```python
from build123d import *

# Parameters (mm, degrees)
F1_W            = 1250
F1_H            = 1250
F2_DEPTH        = 10
F0_W            = 125
F0_H            = 125
F3_DEPTH        = 0.1
F4_W            = 1270
F4_H            = 1270
F4_W_2          = 1250
F4_H_2          = 1250
F5_DEPTH        = 260
F6_W            = 125
F6_H            = 125
F7_DEPTH        = 0.1
F7_COPIES_COUNT = 3
F7_COPIES_ANGLE = 180
F9_W            = 1250
F9_H            = 10
F10_DEPTH       = 250


# Not quite as in the source:
# - a pattern or mirror of a feature is missing from the dataset's text; its kind, count and spacing are read off the source's solid


with BuildPart() as f2:
    # F1 (on Top) → F2 (new body)
    with BuildSketch(Plane.XY):
        Rectangle(F1_W, F1_H)
    extrude(amount=-F2_DEPTH)

    # F0 (on Top) → F3 (cut)
    with BuildSketch(Plane.XY):
        with Locations((-500, 500)):
            Rectangle(F0_W, F0_H)
        with Locations((-250, 500)):
            Rectangle(F0_W, F0_H)
        with Locations((0, 500)):
            Rectangle(F0_W, F0_H)
        with Locations((250, 500)):
            Rectangle(F0_W, F0_H)
        with Locations((500, 500)):
            Rectangle(F0_W, F0_H)
        with Locations((-500, 250)):
            Rectangle(F0_W, F0_H)
        with Locations((-500, 0)):
            Rectangle(F0_W, F0_H)
        with Locations((-500, -250)):
            Rectangle(F0_W, F0_H)
        with Locations((-500, -500)):
            Rectangle(F0_W, F0_H)
        with Locations((250, -500)):
            Rectangle(F0_W, F0_H)
        with Locations((500, -500)):
            Rectangle(F0_W, F0_H)
        with Locations((500, 250)):
            Rectangle(F0_W, F0_H)
        with Locations((-250, -500)):
            Rectangle(F0_W, F0_H)
        with Locations((500, 0)):
            Rectangle(F0_W, F0_H)
        with Locations((0, -500)):
            Rectangle(F0_W, F0_H)
        with Locations((500, -250)):
            Rectangle(F0_W, F0_H)
        Rectangle(F0_W, F0_H)
    extrude(amount=-F3_DEPTH, mode=Mode.SUBTRACT)

    # F4 (on face) → F5 (join)
    with BuildSketch(Plane(origin=(0, 0, -10), x_dir=(1, 0, 0), z_dir=(0, 0, -1))):
        Rectangle(F4_W, F4_H)
        Rectangle(F4_W_2, F4_H_2, mode=Mode.SUBTRACT)
    extrude(amount=-F5_DEPTH)

    # F6 (on face) → F7 (cut)
    with BuildSketch(Plane.YZ.offset(-625)):
        with Locations((-499.9999926, 125.0000074)):
            Rectangle(F6_W, F6_H)
        with Locations((-249.9999926, 125.0000074)):
            Rectangle(F6_W, F6_H)
        with Locations((7.4e-06, 125.0000074)):
            Rectangle(F6_W, F6_H)
        with Locations((250.0000074, 125.0000074)):
            Rectangle(F6_W, F6_H)
        with Locations((500.0000074, 125.0000074)):
            Rectangle(F6_W, F6_H)
    f7 = extrude(amount=-F7_DEPTH, mode=Mode.SUBTRACT)

    # F7_copies: F7 ×3 about axis
    f7_copies_axis = Axis((0, 0, 0), (0, 0, -1))
    for i in range(1, F7_COPIES_COUNT):
        add(f7.rotate(f7_copies_axis, i * F7_COPIES_ANGLE / (F7_COPIES_COUNT - 1)), mode=Mode.SUBTRACT)

    # F9 (on face) → F10 (cut, through all)
    with BuildSketch(Plane.XY.offset(250)):
        with Locations((0, -630)):
            Rectangle(F9_W, F9_H)
    extrude(amount=-F10_DEPTH, mode=Mode.SUBTRACT)


solid = f2.part
```
The listing builds one solid part. Answer for the finished solid, in the listing's coordinates (mm). Give positions to 0.01 mm unless a question says otherwise; leave off trailing zeros. Order: outer loops, then holes, each group sorted by start corner. A loop starts at its lowest first (then second) coordinate and runs counter-clockwise, first axis right, second up. Notation, with made-up numbers: M -32,71 L -9,71 A37 ccw -9,110 Z; hole C -32,66.5 d6. An arc over 180 degrees is marked long. Put each result on its own line as item: value. Start each with the question number.
Item 1: The part is cut by section B-B, the plane y = 31. Determine the outline of the cut face in (x, z).
Item 2: Find the intervals of material crossed by line 1 along X through (y, z) = (155, 175.5); line 2 along X through (y, z) = (-497.5, 96.5); line 3 along Z through (x, y) = (261, -183.5), in increasing order.
Item 3: For a pull along X with two mould halves and no side action, classify faces 1 (the face through (625.1, 1, 126)), 2 (the face through (499, -249, -0.1)), 3 (the face through (635, 9, 118)), 4 (the face through (-3, -635, -6)) as +X half, -X half, draft (parallel to the pull), parting line (faces both ways), or undercut.
Item 4: The part is cut by section D-D, the plane x = 417.5. Determine the outline of the cut face in (y, z).
Item 5: Flat-ended cylindrical pins translate along their axes: P1, Ø12, axis at x = -426, z = 128.5, coming from the -Y side; P2, Ø1, axis at x = -505, y = -355.5, coming from the +Z side. Find the tip coordinate at first contact, or state that the pin passes through.
Item 6: The part is cut by section C-C, the plane y = -232.5. Determine the outline of the cut face in (x, z), and give its area (4 significant figures).
Answer key:
1. outline: M -635,-10 L 635,-10 L 635,250 L 625,250 L 625,187.5 L 625.1,187.5 L 625.1,62.5 L 625,62.5 L 625,0 L 562.5,0 L 562.5,-0.1 L 437.5,-0.1 L 437.5,0 L 62.5,0 L 62.5,-0.1 L -62.5,-0.1 L -62.5,0 L -437.5,0 L -437.5,-0.1 L -562.5,-0.1 L -562.5,0 L -625,0 L -625,62.5 L -625.1,62.5 L -625.1,187.5 L -625,187.5 L -625,250 L -635,250 Z
2. line 1: x = -635 to -625, 625 to 635
2. line 2: x = -635 to -625.1, 625.1 to 635
2. line 3: z = -10 to 0
3. face 1: undercut
3. face 2: undercut
3. face 3: +X half
3. face 4: draft
4. outline: M -635,-10 L 635,-10 L 635,250 L 625,250 L 625,0 L -635,0 Z
5. P1: stops at y = 625
5. P2: stops at z = 0
6. outline: M -635,-10 L 635,-10 L 635,250 L 625,250 L 625,187.5 L 625.1,187.5 L 625.1,62.5 L 625,62.5 L 625,0 L 562.5,0 L 562.5,-0.1 L 437.5,-0.1 L 437.5,0 L -437.5,0 L -437.5,-0.1 L -562.5,-0.1 L -562.5,0 L -625,0 L -625,62.5 L -625.1,62.5 L -625.1,187.5 L -625,187.5 L -625,250 L -635,250 Z
6. area: 17,650 mm²
